The listing builds one solid part. Answer for the finished solid, in the listing's coordinates (mm). Coordinates: 2 decimals unless noted, no trailing zeros. Loops run counter-clockwise (first coordinate to the right, second up) from the corner with the lowest first, then second, coordinate; pieces in that order, holes last. Notation, with made-up numbers: M 58.25,56.25 L 105.25,56.25 A3 cw 105.25,61.25 Z; hole C 37.25,18.5 d3. An arc over 180 degrees is marked long. Answer as a JSON object with one key per item and string values. Group by question number.
1. A cutting plane is placed at C-C on z = 61.5. Give the vertices of the cut face in (x, y).
2. A cutting plane is placed at A-A on z = -38.5. Give the vertices of the cut face in (x, y), and give its area (3 significant figures).
3. A cutting plane is placed at B-B on x = 57.5. Give the vertices of the cut face in (y, z), and give its area (3 significant figures).
4. Straight lines are drawn through the part: L1, parallel to X at y = 3.6, z = -61.5; L2, parallel to Z at x = 82.5, y = 2.2; L3, parallel to X at y = 2.9, z = 38.5. For each, find the intervals that lie inside material, in ascending order.
5. A cutting plane is placed at D-D on y = 2.6. State how many separate pieces and enclosed holes the cut face has, and give its area (3 significant figures).
6. Determine the mould class of faces 1 (the face through (-1, 2, -70)), 2 (the face through (-1, 2, 70)), 3 (the face through (-61.89, 2.54, 20.52)) for opening direction Z: released by +Z, released by -Z, zero draft, split by the parting line, or undercut.
from build123d import *

# Parameters (mm, degrees)
SKETCH1_W   = 180
SKETCH1_H   = 140
BODY_DEPTH  = 5
SKETCH2_R   = 4.5
HOLES_DEPTH = 115.127122105


with BuildPart() as part:
    # Sketch1 → Body (new body)
    with BuildSketch(Plane(origin=(0, 0, 0), x_dir=(1, 0, 0), z_dir=(0, 1, 0))):
        Rectangle(SKETCH1_W, SKETCH1_H)
    extrude(amount=BODY_DEPTH)

    # Sketch2 → Holes (cut, through all)
    with BuildSketch(Plane(origin=(0, 5, 0), x_dir=(1, 0, 0), z_dir=(0, 1, 0))):
        with Locations(Location((-57.5, 61.5, 0), (0, 0, 270))):
            Circle(SKETCH2_R)
        with Locations(Location((-57.5, 38.5, 0), (0, 0, 270))):
            Circle(SKETCH2_R)
        with Locations(Location((-57.5, 1.5, 0), (0, 0, 270))):
            Circle(SKETCH2_R)
        with Locations(Location((-57.5, -21.5, 0), (0, 0, 270))):
            Circle(SKETCH2_R)
        with Locations(Location((-82.5, -38.5, 0), (0, 0, 270))):
            Circle(SKETCH2_R)
        with Locations(Location((-82.5, -61.5, 0), (0, 0, 270))):
            Circle(SKETCH2_R)
        with Locations(Location((-37.5, -61.5, 0), (0, 0, 270))):
            Circle(SKETCH2_R)
        with Locations(Location((-37.5, -38.5, 0), (0, 0, 270))):
            Circle(SKETCH2_R)
        with Locations(Location((37.5, -38.5, 0), (0, 0, 90))):
            Circle(SKETCH2_R)
        with Locations(Location((37.5, -61.5, 0), (0, 0, 90))):
            Circle(SKETCH2_R)
        with Locations(Location((82.5, -61.5, 0), (0, 0, 90))):
            Circle(SKETCH2_R)
        with Locations(Location((82.5, -38.5, 0), (0, 0, 90))):
            Circle(SKETCH2_R)
        with Locations(Location((57.5, -21.5, 0), (0, 0, 90))):
            Circle(SKETCH2_R)
        with Locations(Location((57.5, 1.5, 0), (0, 0, 90))):
            Circle(SKETCH2_R)
        with Locations(Location((57.5, 38.5, 0), (0, 0, 90))):
            Circle(SKETCH2_R)
        with Locations(Location((57.5, 61.5, 0), (0, 0, 90))):
            Circle(SKETCH2_R)
    extrude(amount=-HOLES_DEPTH, mode=Mode.SUBTRACT)


solid = part.part
From the geometry:
{
 "1": {"outline": "M -90,0 L -87,0 L -87,5 L -90,5 Z; M -78,0 L -42,0 L -42,5 L -78,5 Z; M -33,0 L 33,0 L 33,5 L -33,5 Z; M 42,0 L 78,0 L 78,5 L 42,5 Z; M 87,0 L 90,0 L 90,5 L 87,5 Z"},
 "2": {"outline": "M -90,0 L -62,0 L -62,5 L -90,5 Z; M -53,0 L 53,0 L 53,5 L -53,5 Z; M 62,0 L 90,0 L 90,5 L 62,5 Z", "area": "810 mm²"},
 "3": {"outline": "M 0,-70 L 5,-70 L 5,-66 L 0,-66 Z; M 0,-57 L 5,-57 L 5,-43 L 0,-43 Z; M 0,-34 L 5,-34 L 5,-6 L 0,-6 Z; M 0,3 L 5,3 L 5,17 L 0,17 Z; M 0,26 L 5,26 L 5,70 L 0,70 Z", "area": "520 mm²"},
 "4": {"L1": "x = -90 to -62, -53 to 53, 62 to 90", "L2": "z = -70 to 34, 43 to 57, 66 to 70", "L3": "x = -90 to -87, -78 to -42, -33 to 33, 42 to 78, 87 to 90"},
 "5": {"separate pieces": "1", "enclosed holes": "16", "area": "24,200 mm²"},
 "6": {"face 1": "released by -Z", "face 2": "released by +Z", "face 3": "undercut"}
}
